from build123d import *

# Parameters (mm, degrees)
F1_DEPTH = 40
F2_W     = 50
F2_H     = 40
F3_DEPTH = 20


with BuildPart() as f1:
    # F0 (on Front) → F1 (new body)
    with BuildSketch(Plane.XZ):
        with BuildLine():
            Line((25, 0), (25, 50))
            Line((25, 50), (12.5, 50))
            ThreePointArc((12.5, 50), (0, 37.5), (-12.5, 50))
            Line((-12.5, 50), (-25, 50))
            Line((-25, 50), (-25, 0))
            Line((-25, 0), (25, 0))
        make_face()
        with BuildLine():
            Line((12.5, 50), (25, 50))
            ThreePointArc((25, 50), (0, 75), (-25, 50))
            Line((-25, 50), (-12.5, 50))
            ThreePointArc((-12.5, 50), (0, 62.5), (12.5, 50))
        make_face()
    extrude(amount=F1_DEPTH)

    # F2 (on Top) → F3 (join)
    with BuildSketch(Plane.XY):
        with BuildLine():
            Line((-25, 20), (-25, 0))
            Line((-25, 0), (25, 0))
            Line((25, 0), (25, 20))
            Line((25, 20), (12.5, 20))
            ThreePointArc((12.5, 20), (0, 7.5), (-12.5, 20))
            Line((-12.5, 20), (-25, 20))
        make_face()
        with Locations((0, -20)):
            Rectangle(F2_W, F2_H)
        with BuildLine():
            ThreePointArc((25, 20), (0, 45), (-25, 20))
            Line((-25, 20), (-12.5, 20))
            ThreePointArc((-12.5, 20), (0, 32.5), (12.5, 20))
            Line((12.5, 20), (25, 20))
        make_face()
        with BuildLine():
            Line((25, -40), (-25, -40))
            Line((-25, -40), (-25, -60))
            Line((-25, -60), (-12.5, -60))
            ThreePointArc((-12.5, -60), (0, -47.5), (12.5, -60))
            Line((12.5, -60), (25, -60))
            Line((25, -60), (25, -40))
        make_face()
        with BuildLine():
            Line((-12.5, -60), (-25, -60))
            ThreePointArc((-25, -60), (0, -85), (25, -60))
            Line((25, -60), (12.5, -60))
            ThreePointArc((12.5, -60), (0, -72.5), (-12.5, -60))
        make_face()
    extrude(amount=F3_DEPTH)


solid = f1.part
Design review of the part built by this model. Coordinates are the model's own, in mm. A direction names the side the tool comes from. Round coordinates to 2 decimals unless told otherwise and drop trailing zeros. Loops run counter-clockwise (first coordinate to the right, second up) from the corner with the lowest first, then second, coordinate; pieces in that order, holes last. Notation, with made-up numbers: (7.25, -26) - (22.25, -26) arc R7 ccw to (22.25, -14) - close; hole circle Ø11 at (27, 67). An arc over 180 degrees is marked (long way). One line per item, written item: value. Start each with the question number.
1) For faces 4 (the flat face through (0, 0, 36)), 5 (the flat face through (0, -40, 36)), 6 (the cylindrical face through (-5.77, 8.91, 9.86)), list the 3-axis set-ups (+Z, -Z, +X, -X, +Y, -Y) from which the entire face can be reached by the end or side of a thin tool; tool diameter is ignored.
2) Consider section D-D on y = -38.5. Give the boundary of the cut face in (x, z), then the cut area to 3 significant figures.
3) Draft analysis for pull direction Z (two halves, no side actions). For faces 1 (the flat face through (0, -19, 0)), 2 (the cylindrical face through (2.71, -19.72, 37.797)), 3 (the cylindrical face through (-1.627, -72.394, 9.86)), state which applies: +Z half, -Z half, draft (parallel to the pull), parting line (faces both ways), or undercut.
4) Insertion check: pin 1 Ø5 at (x, y) = (-15.5, 32) entering from +Z; pin 2 Ø1.5 at (y, z) = (-17, 60) entering from -X; pin 3 Ø3 at (y, z) = (31, 11) entering from +X. Each pin has a flat end and moves straight along its axis. Give the tip position at first contact, or say it passes through.
5) To check wall thickness, follow L1, parallel to Y at x = 0, z = 4; L2, parallel to X at y = -60, z = 9; L3, parallel to Z at x = 0, y = -13. State the ranges of each line that lie inside material, in increasing order. Write a range as from..to.
6) Consider section C-C on z = 11.5. Give the boundary of the cut face in (x, y), then the cut area to 3 significant figures.
7) Consider section B-B on y = 25. Give the boundary of the cut face in (x, z), then the cut area to 3 significant figures.
8) Consider section A-A on x = 0. Give the boundary of the cut face in (y, z).
Reported:
1. face 4: +Z, +X, -X, +Y
1. face 5: +Z, +X, -X, -Y
1. face 6: +Z, -Z
2. outline: (-25, 0) - (25, 0) - (25, 50) arc R25 ccw to (-25, 50) - close; hole circle Ø25 at (0, 50)
2. area: 2,990 mm^2
3. face 1: -Z half
3. face 2: undercut
3. face 3: draft
4. pin 1: stops at z = 20
4. pin 2: stops at x = -23.23
4. pin 3: stops at x = 23.12
5. L1: y = -85..-72.5, -47.5..7.5, 32.5..45
5. L2: x = -25..-12.5, 12.5..25
5. L3: z = 0..37.5, 62.5..75
6. outline: (-25, -60) arc R25 ccw to (25, -60) - (25, 20) arc R25 ccw to (-25, 20) - close; hole circle Ø25 at (0, -60); hole circle Ø25 at (0, 20)
6. area: 4,980 mm^2
7. outline: (-24.49, 0) - (-11.46, 0) - (-11.46, 20) - (-24.49, 20) - close; (11.46, 0) - (24.49, 0) - (24.49, 20) - (11.46, 20) - close
7. area: 522 mm^2
8. outline: (-85, 0) - (-72.5, 0) - (-72.5, 20) - (-85, 20) - close; (-47.5, 0) - (7.5, 0) - (7.5, 20) - (0, 20) - (0, 37.5) - (-40, 37.5) - (-40, 20) - (-47.5, 20) - close; (-40, 62.5) - (0, 62.5) - (0, 75) - (-40, 75) - close; (32.5, 0) - (45, 0) - (45, 20) - (32.5, 20) - close
